```python
from build123d import *

# Parameters (mm, degrees)
F0_W      = 6.35
F0_H      = 6.477
F1_DEPTH  = 118.11
F2_R      = 1.778
F3_DEPTH  = 25.4
F4_W      = 46.721395
F4_H      = 2.667
F6_DEPTH  = 3.81
F8_DEPTH  = 3.81
F9_DEPTH  = 3.81
F11_DEPTH = 3.81


with BuildPart() as f1:
    # F0 (on Front) → F1 (new body)
    with BuildSketch(Plane.XZ):
        with BuildLine():
            Line((-71.0004344583, -17.2970571), (-23.3659426, -17.2970571))
            Line((-23.3659426, -17.2970571), (23.3659426, 17.2970571))
            Line((23.3659426, 17.2970571), (23.3659426, 23.7740571))
            Line((23.3659426, 23.7740571), (-7.8349318041, 10.194488659))
            ThreePointArc((-7.8349318041, 10.194488659), (-25.7599625829, -12.133990102), (-54.3163019367, -10.0356157532))
            Line((-54.3163019367, -10.0356157532), (-62.6583681975, -13.6663364266))
            Line((-62.6583681975, -13.6663364266), (-86.8754344583, -17.2970571))
            Line((-86.8754344583, -17.2970571), (-71.0004344583, -17.2970571))
        make_face()
        with Locations((26.5409426, 20.5355571)):
            Rectangle(F0_W, F0_H)
    extrude(amount=F1_DEPTH)

    # F2 (on face) → F3 (cut)
    with BuildSketch(Plane.XY.offset(23.7740571)):
        with Locations((26.5409426, -59.055)):
            Circle(F2_R)
        with Locations((26.5409426, -49.6062)):
            Circle(F2_R)
        with Locations((26.5409426, -40.1574)):
            Circle(F2_R)
        with Locations((26.5409426, -68.5038)):
            Circle(F2_R)
        with Locations((26.5409426, -77.9526)):
            Circle(F2_R)
        with Locations((26.5409426, -30.7086)):
            Circle(F2_R)
        with Locations((26.5409426, -87.4014)):
            Circle(F2_R)
    extrude(amount=-F3_DEPTH, mode=Mode.SUBTRACT)

    # F4 (on face) → F5 (join, up to the next surface of F1)
    with BuildSketch(Plane(origin=(0, 0, -17.2970571), x_dir=(1, 0, 0), z_dir=(0, 0, -1))):
        with Locations((-0.0052451, 116.7765)):
            Rectangle(F4_W, F4_H)
        with Locations((-0.0052451, 1.3335)):
            Rectangle(F4_W, F4_H)
    extrude(until=Until.NEXT, dir=(0, 0, 1))

    # F6 (add): a face of the model
    f6_faces = [f1.faces().sort_by_distance(p)[0] for p in [
        (-1.9615853711, -118.11, -2.7916369403),
    ]]
    extrude(f6_faces, amount=F6_DEPTH)

    # F7 (on face) → F8 (join)
    with BuildSketch(Plane.XZ.offset(121.92)):
        with BuildLine():
            Line((-7.8349318041, 10.194488659), (-54.3163019367, -10.0356157532))
            ThreePointArc((-54.3163019367, -10.0356157532), (-25.7599625829, -12.133990102), (-7.8349318041, 10.194488659))
        make_face()
    extrude(amount=-F8_DEPTH)

    # F9 (add): a face of the model
    f9_faces = [f1.faces().sort_by_distance(p)[0] for p in [
        (-1.9615853711, 0, -2.7916369403),
    ]]
    extrude(f9_faces, amount=F9_DEPTH)

    # F10 (on face) → F11 (join)
    with BuildSketch(Plane(origin=(0, 3.81, 0), x_dir=(-1, 0, 0), z_dir=(0, 1, 0))):
        with BuildLine():
            Line((54.3163019367, -10.0356157532), (7.8349318041, 10.194488659))
            ThreePointArc((7.8349318041, 10.194488659), (25.7599625829, -12.133990102), (54.3163019367, -10.0356157532))
        make_face()
    extrude(amount=-F11_DEPTH)


solid = f1.part
```
Verification items for the finished model (mm, model axes). A direction names the side the tool comes from. Round coordinates to 2 decimals unless told otherwise and drop trailing zeros. Order: outer loops, then holes, each group sorted by start corner. A loop starts at its lowest first (then second) coordinate and runs counter-clockwise, first axis right, second up. Notation, with made-up numbers: (79, -38.75) -> (120, -38.75) arc R27 cw to (120, 0.25) -> close; hole circle Ø6 at (70, 63). An arc over 180 degrees is marked (long way). Put each result on its own line as item: value. Start each with the question number.
(1) Depth check by flat-ended pin: pin 1 Ø2 at (x, y) = (26.54, -40.16) entering from -Z; pin 2 Ø6 at (y, z) = (-46.5, -0.5) entering from +X; pin 3 Ø7 at (x, y) = (25, -46) entering from -Z; pin 4 Ø12 at (x, y) = (-39.5, -92) entering from +Z. Enter the tip coordinate at first touch or a pass-through.
(2) Material ranges on line 1 along Y through (x, z) = (18, -14); line 2 along Y through (x, z) = (-38.5, -9.5); line 3 along Z through (x, y) = (-38.5, -35), recorded low to high.
(3) Section check B-B (y = -102). Enter the section's corners in (x, z), then the cut area to 3 significant figures.
(4) Section check A-A (z = -12). Enter the section's corners in (x, y).
(5) Section check C-C (x = -47). Enter the section's corners in (y, z), then the cut area to 3 significant figures.
(6) Draft check along Y on faces 1 (the face through (-57, -60, -17.297)), 2 (the face through (-3, -121.92, -1)), 3 (the face through (-31, -118.11, -5)). Enter one of: +Y half, -Y half, draft (parallel to the pull), parting line (faces both ways), or undercut.
(7) Tool access check on faces 4 (the face through (-25.379, -59.882, -11.965)), 5 (the face through (23.355, 1, 0)), 6 (the face through (-15, 3.81, -6)), 7 (the face through (0, -46, 0)). Record the directions out of +Z, -Z, +X, -X, +Y, -Y that give a thin tool (end or side, any length) a straight path to the whole face; none if there is none.
(8) Section check D-D (z = 6). Enter the section's corners in (x, y), then the cut area to 3 significant figures.
Completed:
1. pin 1: passes through
1. pin 2: stops at x = 3.38
1. pin 3: stops at z = 15.92
1. pin 4: stops at z = -13.77
2. line 1: y = -121.92 to -115.44, -2.67 to 3.81
2. line 2: y = -121.92 to -118.11, 0 to 3.81
2. line 3: z = -17.3 to -14.69
3. outline: (-86.88, -17.3) -> (-23.37, -17.3) -> (23.37, 17.3) -> (29.72, 17.3) -> (29.72, 23.77) -> (23.37, 23.77) -> (-7.83, 10.19) arc R30.78 cw to (-54.32, -10.04) -> (-62.66, -13.67) -> close
3. area: 725 mm2
4. outline: (-58.83, -121.92) -> (23.36, -121.92) -> (23.36, -115.44) -> (-16.21, -115.44) -> (-16.21, -2.67) -> (23.36, -2.67) -> (23.36, 3.81) -> (-58.83, 3.81) -> close; hole (-50.63, -118.11) -> (-25.46, -118.11) -> (-25.46, 0) -> (-50.63, 0) -> close
5. outline: (-121.92, -17.3) -> (3.81, -17.3) -> (3.81, -6.85) -> (0, -6.85) -> (0, -13.36) -> (-118.11, -13.36) -> (-118.11, -6.85) -> (-121.92, -6.85) -> close
5. area: 545 mm2
6. face 1: draft
6. face 2: -Y half
6. face 3: undercut
7. face 4: +Z
7. face 5: -Z, +X, +Y, -Y
7. face 6: +Z, -Z, +X, -X, +Y
7. face 7: -Z, +X
8. outline: (-17.47, -121.92) -> (23.36, -121.92) -> (23.36, -115.44) -> (8.11, -115.44) -> (8.11, -2.67) -> (23.36, -2.67) -> (23.36, 3.81) -> (-17.47, 3.81) -> (-17.47, 0) -> (-8.97, 0) -> (-8.97, -118.11) -> (-17.47, -118.11) -> close
8. area: 2,410 mm2
